Geometry: final body of the model. Coordinates: model frame, mm. Give positions to 0.01 mm unless a question says otherwise; leave off trailing zeros. Write each loop counter-clockwise with the first axis right and the second up, starting at its lowest first coordinate (ties: lowest second). Pieces come first, ordered by that corner, then holes.
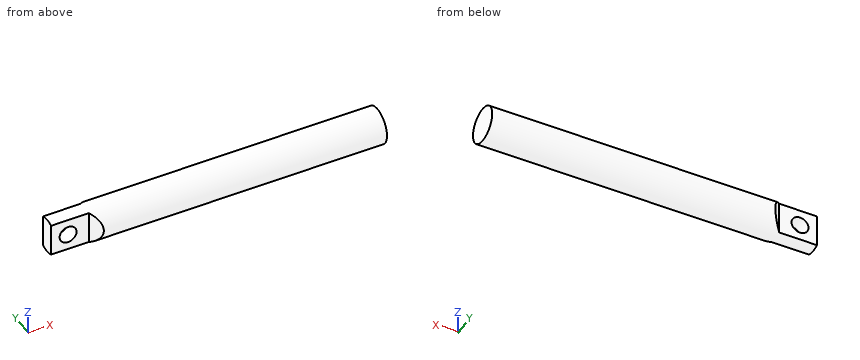
```python
from build123d import *

# Parameters (mm, degrees)
SKETCH1_R               = 9.5
BOSS_EXTRUDE1_DEPTH     = 175
CUT_EXTRUDE1_DEPTH      = 176.514956628
CUT_EXTRUDE1_DEPTH_BACK = 176.514956628
SKETCH4_R               = 4.5
CUT_EXTRUDE2_DEPTH      = 176.776847167


with BuildPart() as part:
    # Sketch1 → Boss-Extrude1 (new body)
    with BuildSketch(Plane(origin=(0, 0, 0), x_dir=(0, 0, -1), z_dir=(1, 0, 0))):
        Circle(SKETCH1_R)
    extrude(amount=BOSS_EXTRUDE1_DEPTH)

    # Sketch3 → Cut-Extrude1 (cut, two sides: drawn at the far end of the back side and taken through both)
    with BuildSketch(Plane.XY.offset(-CUT_EXTRUDE1_DEPTH_BACK)):
        Polygon((20, 4), (0, 4), (0, 9.5), (25, 9.5), align=None)
        Polygon((20, -4), (0, -4), (0, -9.5), (25, -9.5), align=None)
    extrude(amount=CUT_EXTRUDE1_DEPTH + CUT_EXTRUDE1_DEPTH_BACK, mode=Mode.SUBTRACT)

    # Sketch4 → Cut-Extrude2 (cut, through all)
    with BuildSketch(Plane(origin=(0, 4, 0), x_dir=(1, 0, 0), z_dir=(0, 1, 0))):
        with Locations(Location((9, 0, 0), (0, 0, 270))):
            Circle(SKETCH4_R)
    extrude(amount=-CUT_EXTRUDE2_DEPTH, mode=Mode.SUBTRACT)


solid = part.part
```
Item 1: Section D-D, the plane x = 134. Return the cut outline in (y, z), plus the area to 3 significant figures.
Found:
outline: circle Ø19 at (0, 0)
area: 284 mm2
Item 2: Section B-B, the plane x = 9. Return the cut outline in (y, z), plus the area to 3 significant figures.
Found:
outline: (-4, -8.62) arc R9.5 ccw to (4, -8.62) - (4, -4.5) - (-4, -4.5) - close; (-4, 4.5) - (4, 4.5) - (4, 8.62) arc R9.5 ccw to (-4, 8.62) - close
area: 75.4 mm2
Item 3: Section C-C, the plane y = 0. Return the cut outline in (x, z).
Found:
outline: (0, -9.5) - (175, -9.5) - (175, 9.5) - (0, 9.5) - close; hole circle Ø9 at (9, 0)
Item 4: Section A-A, the plane z = 0. Return the cut outline in (x, y), plus the area to 3 significant figures.
Found:
outline: (0, -4) - (4.5, -4) - (4.5, 4) - (0, 4) - close; (13.5, -4) - (20, -4) - (25, -9.5) - (175, -9.5) - (175, 9.5) - (25, 9.5) - (20, 4) - (13.5, 4) - close
area: 3,010 mm2
Item 5: Pin query (flat end, axial travel): pin 1 Ø3 at (y, z) = (4.5, 1.5) entering from -X; pin 2 Ø5 at (x, z) = (13, 2) entering from +Y; pin 3 Ø5 at (x, z) = (115, 4.5) entering from -Y; pin 4 Ø5 at (x, z) = (14, 1.5) entering from -Y. Return the tip coordinate at first contact, or that it passes through.
Found:
pin 1: stops at x = 0
pin 2: stops at y = 4
pin 3: stops at y = -9.29
pin 4: stops at y = -4
Item 6: Line query: L1, parallel to X at y = 2.5, z = 0; L2, parallel to Y at x = 42, z = 0.5. Output: solid intervals per line, ascending.
Found:
L1: x = 0 to 4.5, 13.5 to 175
L2: y = -9.49 to 9.49
